Part model, mm, in its own coordinate system. Coordinates: 2 decimals unless noted, no trailing zeros. Order: outer loops, then holes, each group sorted by start corner. A loop starts at its lowest first (then second) coordinate and runs counter-clockwise, first axis right, second up.
1) Cut at D-D (z = 11). List the corners of the cut face in (x, y).
2) Cut at B-B (z = 0). Give the number of separate pieces and of enclosed holes in the cut face, and give its area (3 significant figures).
3) Cut at A-A (x = 0). List the corners of the cut face in (y, z), and give its area (3 significant figures).
4) Wall check: L1, parallel to Z at x = -44, y = 3.6; L2, parallel to Z at x = -36.5, y = 1.6; L3, parallel to X at y = 2.35, z = -31. Give the ranges that are in metal, low to high.
5) Mould opens along X. For faces 1 (the flat face through (59, 2, 31)), 2 (the flat face through (-25, 0, 0)), 3 (the cylindrical face through (-26.829, 2.028, -9.776)), 4 (the flat face through (-56, 2, 0)) say: +X half, -X half, draft (parallel to the pull), parting line (faces both ways), or undercut.
6) Cut at C-C (x = -42). List the corners of the cut face in (y, z), and give its area (3 significant figures).
7) Pin check, flat tips, straight feed: pin 1 Ø3 at (x, z) = (42, 7) entering from -Y; pin 2 Ø2 at (y, z) = (2, -9) entering from +X; pin 3 Ø0.5 at (x, y) = (57.5, 2.5) entering from -Z. Stop position of each tip, or through.
```python
from build123d import *

# Parameters (mm, degrees)
SKETCH_1_W          = 112
SKETCH_1_H          = 70
SKETCH_1_W_2        = 3
SKETCH_1_H_2        = 40
EXTRUDE_1_DEPTH     = 4
SKETCH_6_R          = 21.5
SKETCH_6_R_2        = 2
CUT_EXTRUDE_5_DEPTH = 67.158899628
SKETCH_2_R          = 1.5
CUT_EXTRUDE_1_DEPTH = 10
SKETCH_4_R          = 1
CUT_EXTRUDE_3_DEPTH = 67.158899628
CUT_EXTRUDE_6_DEPTH = 67.158899628
SKETCH_8_W          = 3
SKETCH_8_H          = 8
EXTRUDE_2_DEPTH     = 4
SKETCH_9_R          = 1.5
CUT_EXTRUDE_7_DEPTH = 69.71681017
FILLET_3_R          = 1


with BuildPart() as part:
    # 草图1 → 凸台-拉伸1 (new body)
    with BuildSketch(Plane(origin=(0, 0, 0), x_dir=(1, 0, 0), z_dir=(0, 1, 0))):
        Rectangle(SKETCH_1_W, SKETCH_1_H)
        with Locations((-51.5, 0)):
            Rectangle(SKETCH_1_W_2, SKETCH_1_H_2, mode=Mode.SUBTRACT)
        with Locations((51.5, 0)):
            Rectangle(SKETCH_1_W_2, SKETCH_1_H_2, mode=Mode.SUBTRACT)
    extrude(amount=EXTRUDE_1_DEPTH)

    # 草图6 → 切除-拉伸5 (cut, through all)
    with BuildSketch(Plane(origin=(0, 4, 0), x_dir=(1, 0, 0), z_dir=(0, 1, 0))):
        with Locations(Location((0, 0, 0), (0, 0, 270))):
            Circle(SKETCH_6_R)
        with Locations(Location((-25.980762114, 15, 0), (0, 0, 270))):
            Circle(SKETCH_6_R_2)
        with Locations(Location((25.980762114, 15, 0), (0, 0, 270))):
            Circle(SKETCH_6_R_2)
        with Locations(Location((0, -30, 0), (0, 0, 270))):
            Circle(SKETCH_6_R_2)
        with BuildLine():
            ThreePointArc((-29.943700615, 8.023390398), (-31, 0), (-29.943700615, -8.023390398))
            ThreePointArc((-29.943700615, -8.023390398), (-26.881838436, -9.791157351), (-25.114071484, -6.729295173))
            ThreePointArc((-25.114071484, -6.729295173), (-26, 0), (-25.114071484, 6.729295173))
            ThreePointArc((-25.114071484, 6.729295173), (-26.881838436, 9.791157351), (-29.943700615, 8.023390398))
        make_face()
        with BuildLine():
            ThreePointArc((29.943700615, 8.023390398), (31, 0), (29.943700615, -8.023390398))
            ThreePointArc((29.943700615, -8.023390398), (26.881838436, -9.791157351), (25.114071484, -6.729295173))
            ThreePointArc((25.114071484, -6.729295173), (26, 0), (25.114071484, 6.729295173))
            ThreePointArc((25.114071484, 6.729295173), (26.881838436, 9.791157351), (29.943700615, 8.023390398))
        make_face()
    extrude(amount=-CUT_EXTRUDE_5_DEPTH, mode=Mode.SUBTRACT)

    # 草图2 → 切除-拉伸1 (cut)
    with BuildSketch(Plane(origin=(0, 4, 0), x_dir=(1, 0, 0), z_dir=(0, 1, 0))):
        with Locations(Location((-47, 31, 0), (0, 0, 270))):
            Circle(SKETCH_2_R)
        with Locations(Location((47, 31, 0), (0, 0, 270))):
            Circle(SKETCH_2_R)
        with Locations(Location((47, -31, 0), (0, 0, 270))):
            Circle(SKETCH_2_R)
        with Locations(Location((-47, -31, 0), (0, 0, 270))):
            Circle(SKETCH_2_R)
    extrude(amount=-CUT_EXTRUDE_1_DEPTH, mode=Mode.SUBTRACT)

    # 草图4 → 切除-拉伸3 (cut, through all)
    with BuildSketch(Plane.XZ.offset(-4)):
        with Locations((-50, 19)):
            Circle(SKETCH_4_R)
        with Locations((-50, -19)):
            Circle(SKETCH_4_R)
        with Locations((50, -19)):
            Circle(SKETCH_4_R)
        with Locations((50, 19)):
            Circle(SKETCH_4_R)
        with Locations((-53, 19)):
            Circle(SKETCH_4_R)
        with Locations((-53, -19)):
            Circle(SKETCH_4_R)
        with Locations((53, -19)):
            Circle(SKETCH_4_R)
        with Locations((53, 19)):
            Circle(SKETCH_4_R)
    extrude(amount=CUT_EXTRUDE_3_DEPTH, mode=Mode.SUBTRACT)

    # 草图7 → 切除-拉伸6 (cut, through all)
    with BuildSketch(Plane(origin=(0, 4, 0), x_dir=(1, 0, 0), z_dir=(0, 1, 0))):
        with BuildLine():
            Line((-28.618176043, 25), (-45, 25))
            Line((-45, 25), (-45, 14))
            Line((-45, 14), (-35.327043465, 14))
            ThreePointArc((-35.327043465, 14), (-32.442222095, 19.786415176), (-28.618176043, 25))
        make_face()
        with BuildLine():
            Line((-36.918829884, 9), (-45, 9))
            Line((-45, 9), (-45, -9))
            Line((-45, -9), (-36.918829884, -9))
            ThreePointArc((-36.918829884, -9), (-38, 0), (-36.918829884, 9))
        make_face()
        with BuildLine():
            Line((-45, -14), (-35.327043465, -14))
            ThreePointArc((-35.327043465, -14), (-32.442222095, -19.786415176), (-28.618176043, -25))
            Line((-28.618176043, -25), (-45, -25))
            Line((-45, -25), (-45, -14))
        make_face()
        with BuildLine():
            Line((28.618176043, -25), (45, -25))
            Line((45, -25), (45, -14))
            Line((45, -14), (35.327043465, -14))
            ThreePointArc((35.327043465, -14), (32.442222095, -19.786415176), (28.618176043, -25))
        make_face()
        with BuildLine():
            Line((36.918829884, -9), (45, -9))
            Line((45, -9), (45, 9))
            Line((45, 9), (36.918829884, 9))
            ThreePointArc((36.918829884, 9), (38, 0), (36.918829884, -9))
        make_face()
        with BuildLine():
            Line((45, 14), (35.327043465, 14))
            ThreePointArc((35.327043465, 14), (32.442222095, 19.786415176), (28.618176043, 25))
            Line((28.618176043, 25), (45, 25))
            Line((45, 25), (45, 14))
        make_face()
    extrude(amount=-CUT_EXTRUDE_6_DEPTH, mode=Mode.SUBTRACT)

    # 草图8 → 凸台-拉伸2 (add)
    with BuildSketch(Plane(origin=(0, 4, 0), x_dir=(1, 0, 0), z_dir=(0, 1, 0))):
        with Locations((57.5, -31)):
            Rectangle(SKETCH_8_W, SKETCH_8_H)
    extrude(amount=-EXTRUDE_2_DEPTH)

    # 草图9 → 切除-拉伸7 (cut, through all)
    with BuildSketch(Plane(origin=(0, 4, 0), x_dir=(1, 0, 0), z_dir=(0, 1, 0))):
        with Locations(Location((56, -31, 0), (0, 0, 270))):
            Circle(SKETCH_9_R)
    extrude(amount=-CUT_EXTRUDE_7_DEPTH, mode=Mode.SUBTRACT)

    # 圆角3
    fillet_3_edges = [part.edges().sort_by_distance(p)[0] for p in [
        (35.327043465, 2, -14),
        (28.618176043, 2, -25),
        (45, 2, -25),
        (45, 2, -14),
        (36.918829884, 2, 9),
        (36.918829884, 2, -9),
        (45, 2, -9),
        (45, 2, 9),
        (28.618176043, 2, 25),
        (35.327043465, 2, 14),
        (45, 2, 14),
        (45, 2, 25),
        (-35.327043465, 2, 14),
        (-28.618176043, 2, 25),
        (-45, 2, 25),
        (-45, 2, 14),
        (-36.918829884, 2, -9),
        (-36.918829884, 2, 9),
        (-28.618176043, 2, -25),
        (-35.327043465, 2, -14),
        (-45, 2, -14),
        (-45, 2, -25),
        (56, 2, 27),
        (59, 2, 27),
        (59, 2, 35),
        (-56, 2, -35),
        (56, 2, -35),
        (-56, 2, 35),
    ]]
    fillet(fillet_3_edges, radius=FILLET_3_R)


solid = part.part
```
Geometry check:
1. outline: (-56, 0) - (-53, 0) - (-53, 4) - (-56, 4) - close; (-50, 0) - (-18.47, 0) - (-18.47, 4) - (-50, 4) - close; (18.47, 0) - (50, 0) - (50, 4) - (18.47, 4) - close; (53, 0) - (56, 0) - (56, 4) - (53, 4) - close
2. separate pieces: 8
2. enclosed holes: 0
2. area: 156 mm2
3. outline: (0, -35) - (4, -35) - (4, -21.5) - (0, -21.5) - close; (0, 21.5) - (4, 21.5) - (4, 28) - (0, 28) - close; (0, 32) - (4, 32) - (4, 35) - (0, 35) - close
3. area: 92.0 mm2
4. L1: z = -35 to -25, -14 to -9, 9 to 14, 25 to 35
4. L2: z = -35 to -25, -14 to 14, 25 to 35
4. L3: x = -56 to -48.5, -45.5 to 45.5, 48.5 to 56
5. face 1: +X half
5. face 2: draft
5. face 3: undercut
5. face 4: -X half
6. outline: (0, -35) - (4, -35) - (4, -25) - (0, -25) - close; (0, -14) - (4, -14) - (4, -9) - (0, -9) - close; (0, 9) - (4, 9) - (4, 14) - (0, 14) - close; (0, 25) - (4, 25) - (4, 35) - (0, 35) - close
6. area: 120 mm2
7. pin 1: passes through
7. pin 2: stops at x = 56
7. pin 3: stops at z = 27
